Design review of the part built by this model. Coordinates are the model's own, in mm. Face numbers are marked on the shaded views. A direction names the side the tool comes from. Coordinates: 2 decimals unless noted, no trailing zeros. Write each loop counter-clockwise with the first axis right and the second up, starting at its lowest first coordinate (ties: lowest second). Pieces come first, ordered by that corner, then holes.
Q1. Take a section at C-C (x = 0). Give the boundary of the cut face in (y, z), and give its area (3 significant figures).
Q2. Insertion check: pin 1 (3 mm diameter, centred on x = -9.5, z = 0, fed in from +Y); pin 2 (8 mm diameter, centred on y = 14, z = 6, fed in from +X); pin 3 (4 mm diameter, centred on y = 24, z = 10, fed in from +X). Each pin has a flat end and moves straight along its axis. Give the tip position at first contact, or say it passes through.
Q3. Mouldability with a two-part tool opening along X and no side actions: class the marked faces 3, 4, 5 and 6 as pulls with the +X half, pulls with the -X half, needs draft (parallel to the pull), parting line crosses it, or undercut.
Q4. Take a section at B-B (z = 0). Give the boundary of the cut face in (x, y), and give its area (3 significant figures).
Q5. Machinability: for the marked faces 1 and 2, which of the approach directions +Z, -Z, +X, -X, +Y, -Y give a long, thin tool a straight path to every point of the face, cutting with its end or side? Answer none if there is none.
Q6. Take a section at D-D (y = 15). Give the boundary of the cut face in (x, z), and give its area (3 significant figures).
Q7. For probe 1 along Z at (x, y) = (0, 27); probe 2 along X at (y, z) = (6, -0.5); probe 3 along Y at (x, z) = (20, 3.5), list the stretches that pass through material, from the lowest coordinate up.
Q8. Take a section at A-A (y = 26). Give the boundary of the cut face in (x, z), and give its area (3 significant figures).
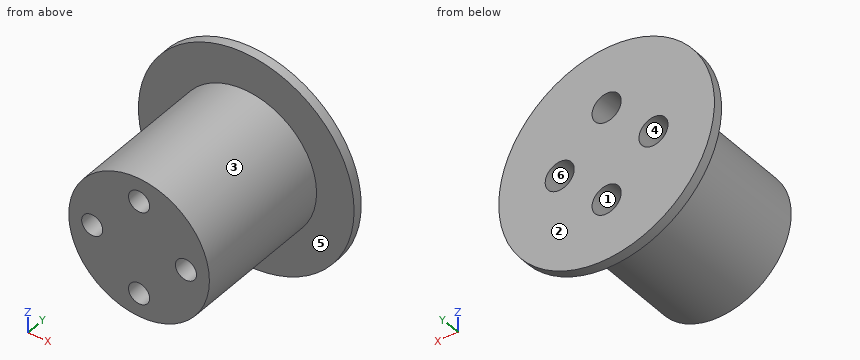
```python
from build123d import *

# Parameters (mm, degrees)
SKETCH1_R           = 15
BOSS_EXTRUDE1_DEPTH = 30
SKETCH2_R           = 23
BOSS_EXTRUDE2_DEPTH = 2
SKETCH3_R           = 2.25
CUT_EXTRUDE1_DEPTH  = 10
SKETCH4_R           = 3.1
CUT_EXTRUDE2_DEPTH  = 10


with BuildPart() as part:
    # Sketch1 → Boss-Extrude1 (new body)
    with BuildSketch(Plane(origin=(0, 0, 0), x_dir=(1, 0, 0), z_dir=(0, 1, 0))):
        Circle(SKETCH1_R)
    extrude(amount=BOSS_EXTRUDE1_DEPTH)

    # Sketch2 → Boss-Extrude2 (add)
    with BuildSketch(Plane(origin=(0, 30, 0), x_dir=(1, 0, 0), z_dir=(0, 1, 0))):
        Circle(SKETCH2_R)
    extrude(amount=BOSS_EXTRUDE2_DEPTH)

    # Sketch3 → Cut-Extrude1 (cut)
    with BuildSketch(Plane.XZ):
        with Locations((0, 10)):
            Circle(SKETCH3_R)
        with Locations((10, 0)):
            Circle(SKETCH3_R)
        with Locations((0, -10)):
            Circle(SKETCH3_R)
        with Locations((-10, 0)):
            Circle(SKETCH3_R)
    extrude(amount=-CUT_EXTRUDE1_DEPTH, mode=Mode.SUBTRACT)

    # Sketch4 → Cut-Extrude2 (cut)
    with BuildSketch(Plane(origin=(0, 32, 0), x_dir=(1, 0, 0), z_dir=(0, 1, 0))):
        with Locations((0, 10)):
            Circle(SKETCH4_R)
        with Locations((10, 0)):
            Circle(SKETCH4_R)
        with Locations((0, -10)):
            Circle(SKETCH4_R)
        with Locations((-10, 0)):
            Circle(SKETCH4_R)
    extrude(amount=-CUT_EXTRUDE2_DEPTH, mode=Mode.SUBTRACT)


solid = part.part
```
Response:
1. outline: (0, -15) - (30, -15) - (30, -23) - (32, -23) - (32, -13.1) - (22, -13.1) - (22, -6.9) - (32, -6.9) - (32, 6.9) - (22, 6.9) - (22, 13.1) - (32, 13.1) - (32, 23) - (30, 23) - (30, 15) - (0, 15) - (0, 12.25) - (10, 12.25) - (10, 7.75) - (0, 7.75) - (0, -7.75) - (10, -7.75) - (10, -12.25) - (0, -12.25) - close
1. area: 778 mm2
2. pin 1: stops at y = 22
2. pin 2: stops at x = 14.87
2. pin 3: stops at x = 12.69
3. face 3: parting line crosses it
3. face 4: undercut
3. face 5: needs draft
3. face 6: undercut
4. outline: (-23, 30) - (-15, 30) - (-15, 0) - (-12.25, 0) - (-12.25, 10) - (-7.75, 10) - (-7.75, 0) - (7.75, 0) - (7.75, 10) - (12.25, 10) - (12.25, 0) - (15, 0) - (15, 30) - (23, 30) - (23, 32) - (13.1, 32) - (13.1, 22) - (6.9, 22) - (6.9, 32) - (-6.9, 32) - (-6.9, 22) - (-13.1, 22) - (-13.1, 32) - (-23, 32) - close
4. area: 778 mm2
5. face 1: +Y
5. face 2: +Z, -Z, +X, -X, +Y
6. outline: circle Ø30 at (0, 0)
6. area: 707 mm2
7. probe 1: z = -15 to -13.1, -6.9 to 6.9, 13.1 to 15
7. probe 2: x = -14.99 to -12.19, -7.81 to 7.81, 12.19 to 14.99
7. probe 3: y = 30 to 32
8. outline: circle Ø30 at (0, 0); hole circle Ø6.2 at (-10, 0); hole circle Ø6.2 at (0, -10); hole circle Ø6.2 at (0, 10); hole circle Ø6.2 at (10, 0)
8. area: 586 mm2
